Part model, mm, in its own coordinate system. A direction names the side the tool comes from. Coordinates: 2 decimals unless noted, no trailing zeros. Loops run counter-clockwise (first coordinate to the right, second up) from the corner with the lowest first, then second, coordinate; pieces in that order, holes last. Notation, with made-up numbers: (89.5, -6) - (118.5, -6) arc R27 ccw to (118.5, 22) - close; hole circle Ø8 at (28, 86). An arc over 180 degrees is marked (long way). Use a Markdown table: item, result. Add a question column.
1) Tool access for faces 1 (the face through (-5.5, 0, 1)), 2 (the face through (-15, -8, 2)): list every direction of +Z, -Z, +X, -X, +Y, -Y with a clear straight run to the whole face (end or side of a thin tool).
2) Pull direction Y, two halves, no side cores. Call faces 3 (the face through (2, -22, -1)), 4 (the face through (-25, 17.57, 0.99)), 5 (the face through (21, 3, 2)), 6 (the face through (-25.07, -17.5, 0.99)): +Y half, -Y half, draft (parallel to the pull), parting line (faces both ways), or undercut.
3) Band-saw the part on B-B (x = 0.5). Give the cut face in (y, z), plus the area to 3 significant figures.
4) Band-saw the part on D-D (y = 12). Give the cut face in (x, z).
5) Band-saw the part on C-C (x = 17.5). Give the cut face in (y, z).
6) Band-saw the part on A-A (z = -1). Give the cut face in (x, y).
7) Probe probe 1 along X at (y, z) = (0, -1.95); probe 2 along Y at (x, z) = (-11.5, 0.85); probe 3 along Y at (x, z) = (17.5, -0.9). List the from-to ranges inside material, lowest first. Write a range as [from, to].
8) Drop a flat-ended pin along its axis: P1, Ø1.5, axis at y = -16, z = -2, coming from the -X side. Give the stop position or say it passes through.
from build123d import *

# Parameters (mm, degrees)
PAD_DEPTH        = 3
PAD001_DEPTH     = 2
HOLE_D           = 5
HOLE_DEPTH       = 25
HOLE_CSINK_D     = 8
HOLE_CSINK_ANGLE = 90


with BuildPart() as part:
    # Sketch001 → Pad (new body)
    with BuildSketch(Plane.XY):
        with BuildLine():
            ThreePointArc((-21.5, 22), (-27.156854, 19.656854), (-29.5, 14))
            Line((-29.5, -14), (-29.5, 14))
            ThreePointArc((-29.5, -14), (-27.156854, -19.656854), (-21.5, -22))
            Line((24.5, -22), (-21.5, -22))
            ThreePointArc((24.5, -22), (30.156854, -19.656854), (32.5, -14))
            Line((32.5, 14), (32.5, -14))
            ThreePointArc((32.5, 14), (30.156854, 19.656854), (24.5, 22))
            Line((-21.5, 22), (24.5, 22))
        make_face()
    extrude(amount=-PAD_DEPTH)

    # Sketch → Pad001 (join)
    with BuildSketch(Plane.XY):
        with BuildLine():
            ThreePointArc((-21.5, 22), (-27.156854, 19.656854), (-29.5, 14))
            Line((-29.5, -14), (-29.5, 14))
            ThreePointArc((-29.5, -14), (-27.156854, -19.656854), (-21.5, -22))
            Line((24.5, -22), (-21.5, -22))
            ThreePointArc((24.5, -22), (30.156854, -19.656854), (32.5, -14))
            Line((32.5, 14), (32.5, -14))
            ThreePointArc((32.5, 14), (30.156854, 19.656854), (24.5, 22))
            Line((-21.5, 22), (24.5, 22))
        make_face()
        with BuildLine():
            ThreePointArc((-26.5, -14), (-25.035534, -17.535534), (-21.5, -19))
            Line((24.5, -19), (-21.5, -19))
            ThreePointArc((24.5, -19), (28.035534, -17.535534), (29.5, -14))
            Line((29.5, 14), (29.5, -14))
            ThreePointArc((29.5, 14), (28.035534, 17.535534), (24.5, 19))
            Line((-21.5, 19), (24.5, 19))
            ThreePointArc((-21.5, 19), (-25.035534, 17.535534), (-26.5, 14))
            Line((-26.5, -14), (-26.5, 14))
        make_face(mode=Mode.SUBTRACT)
        Polygon((-21.5, 14), (-21.5, -14), (-7.5, -14), (-7.5, -6), (-13.5, -6), (-13.5, 14), align=None)
        Polygon((8.5, 14), (-5.5, 14), (-5.5, -14), (8.5, -14), (8.5, -6), (2.5, -6), (2.5, -4), (6.5, -4), (6.5, 4), (2.5, 4), (2.5, 6), (8.5, 6), align=None)
        with BuildLine():
            Line((13.5, 14), (21.5, 14))
            ThreePointArc((24.5, 11), (23.62132, 13.12132), (21.5, 14))
            Line((24.5, 11), (24.5, -11))
            ThreePointArc((21.5, -14), (23.62132, -13.12132), (24.5, -11))
            Line((21.5, -14), (13.5, -14))
            ThreePointArc((10.5, -11), (11.37868, -13.12132), (13.5, -14))
            Line((10.5, -11), (10.5, 11))
            ThreePointArc((13.5, 14), (11.37868, 13.12132), (10.5, 11))
        make_face()
    extrude(amount=PAD001_DEPTH)

    # Hole
    with Locations(Plane.XY.offset(2)):
        with Locations((-17.5, 0), (17.5, 0)):
            CounterSinkHole(HOLE_D / 2, HOLE_CSINK_D / 2, depth=HOLE_DEPTH, counter_sink_angle=HOLE_CSINK_ANGLE)


solid = part.part
Answer block:
| question | item | result |
|---|---|---|
| 1 | face 1 | +Z |
| 1 | face 2 | +Z, +X, -X, +Y, -Y |
| 2 | face 3 | -Y half |
| 2 | face 4 | undercut |
| 2 | face 5 | draft |
| 2 | face 6 | undercut |
| 3 | outline | (-22, -3) - (22, -3) - (22, 2) - (19, 2) - (19, 0) - (14, 0) - (14, 2) - (-14, 2) - (-14, 0) - (-19, 0) - (-19, 2) - (-22, 2) - close |
| 3 | area | 200 mm2 |
| 4 | outline | (-29.5, -3) - (32.5, -3) - (32.5, 2) - (29.5, 2) - (29.5, 0) - (24.33, 0) - (24.33, 2) - (10.67, 2) - (10.67, 0) - (8.5, 0) - (8.5, 2) - (-5.5, 2) - (-5.5, 0) - (-13.5, 0) - (-13.5, 2) - (-21.5, 2) - (-21.5, 0) - (-26.5, 0) - (-26.5, 2) - (-29.5, 2) - close |
| 5 | outline | (-22, -3) - (-2.5, -3) - (-2.5, 0.5) - (-4, 2) - (-14, 2) - (-14, 0) - (-19, 0) - (-19, 2) - (-22, 2) - close; (2.5, -3) - (22, -3) - (22, 2) - (19, 2) - (19, 0) - (14, 0) - (14, 2) - (4, 2) - (2.5, 0.5) - close |
| 6 | outline | (-29.5, -14) arc R8 ccw to (-21.5, -22) - (24.5, -22) arc R8 ccw to (32.5, -14) - (32.5, 14) arc R8 ccw to (24.5, 22) - (-21.5, 22) arc R8 ccw to (-29.5, 14) - close; hole circle Ø5 at (-17.5, 0); hole circle Ø5 at (17.5, 0) |
| 7 | probe 1 | [-29.5, -20], [-15, 15], [20, 32.5] |
| 7 | probe 2 | [-22, -19], [-14, -6], [19, 22] |
| 7 | probe 3 | [-22, -2.5], [2.5, 22] |
| 8 | P1 | x = -29.4 |
